Build history of the part. All positions in model axes, mm. Face numbers are marked on the shaded views. A direction names the side the tool comes from. Give positions to 0.01 mm unless a question says otherwise; leave off trailing zeros. Write each loop counter-clockwise with the first axis right and the second up, starting at its lowest first coordinate (ties: lowest second). Pieces come first, ordered by that corner, then holes. Notation, with made-up numbers: (78.25, 6.5) -> (133.25, 6.5) arc R14 ccw to (133.25, 12.5) -> close; hole circle Ø1 at (-18, 10). An arc over 180 degrees is marked (long way). One line per question, with ' | ' between items. Start each with the question number.
(1) Band-saw the part on C-C, the plane z = -3. Give the cut face in (x, y), and give its area (3 significant figures).
(2) Drill centre lines: probe 1 along X at (y, z) = (2.5, -2.25); probe 2 along X at (y, z) = (-2.5, -10.5). Where is each one in solid material? Low to high. Write a range as from..to.
(3) Band-saw the part on D-D, the plane x = 1.75. Give the cut face in (y, z).
(4) Band-saw the part on B-B, the plane y = 0. Give the cut face in (x, z).
(5) Band-saw the part on A-A, the plane x = 0. Give the cut face in (y, z), and give its area (3 significant figures).
(6) Tool access for the marked faces 1, 2 and 3: list every direction of +Z, -Z, +X, -X, +Y, -Y with a clear straight run to the whole face (end or side of a thin tool).
(7) Pin check, flat tips, straight feed: P1, Ø2, axis at x = -2.5, z = -8, coming from the +Y side; P2, Ø2, axis at x = -2, z = -9, coming from the -Y side; P3, Ø3, axis at x = 1, y = -1.5, coming from the -Z side. Stop position of each tip, or through.
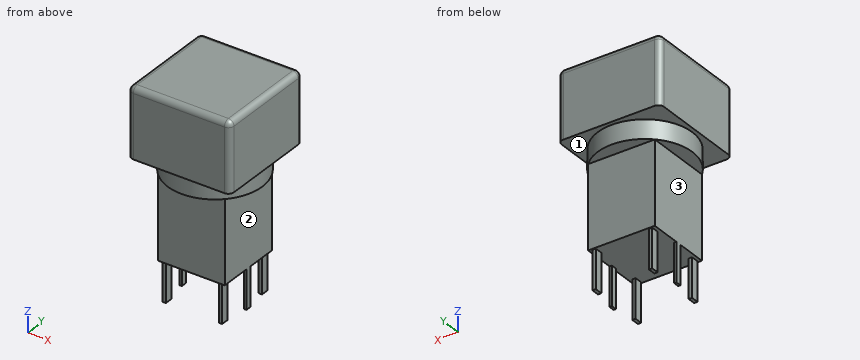
from build123d import *

# Parameters (mm, degrees)
SKETCH_1_W      = 9.2
SKETCH_1_H      = 9.2
EXTRUDE_1_DEPTH = 6.2
FILLET_1_R      = 0.5
SKETCH_2_R      = 4.25
EXTRUDE_2_DEPTH = 1.7
SKETCH_3_W      = 6
SKETCH_3_H      = 6
EXTRUDE_3_DEPTH = 7.45
SKETCH_4_W      = 0.3
SKETCH_4_H      = 0.7
SKETCH_4_W_2    = 0.2
SKETCH_4_H_2    = 0.5
EXTRUDE_4_DEPTH = 3.5


with BuildPart() as part:
    # Эскиз1 → Бобышка-Вытянуть1 (new body)
    with BuildSketch(Plane.XY):
        Rectangle(SKETCH_1_W, SKETCH_1_H)
    extrude(amount=EXTRUDE_1_DEPTH)

    # Скругление1
    fillet_1_edges = [part.edges().sort_by_distance(p)[0] for p in [
        (-4.6, 0, 6.2),
        (0, -4.6, 6.2),
        (4.6, 0, 6.2),
        (4.6, -4.6, 3.1),
        (-4.6, -4.6, 3.1),
        (-4.6, 4.6, 3.1),
        (4.6, 4.6, 3.1),
        (0, 4.6, 6.2),
    ]]
    fillet(fillet_1_edges, radius=FILLET_1_R)

    # Эскиз2 → Бобышка-Вытянуть2 (add)
    with BuildSketch(Plane(origin=(0, 0, 0), x_dir=(-1, 0, 0), z_dir=(0, 0, -1))):
        Circle(SKETCH_2_R)
    extrude(amount=EXTRUDE_2_DEPTH)

    # Эскиз3 → Бобышка-Вытянуть3 (add)
    with BuildSketch(Plane(origin=(0, 0, -1.7), x_dir=(-1, 0, 0), z_dir=(0, 0, -1))):
        Rectangle(SKETCH_3_W, SKETCH_3_H)
    extrude(amount=EXTRUDE_3_DEPTH)

    # Эскиз4 → Бобышка-Вытянуть4 (add)
    with BuildSketch(Plane(origin=(0, 0, -9.15), x_dir=(-1, 0, 0), z_dir=(0, 0, -1))):
        with Locations((-2.54, 2.54)):
            Rectangle(SKETCH_4_W, SKETCH_4_H)
        with Locations((2.54, 2.54)):
            Rectangle(SKETCH_4_W, SKETCH_4_H)
        with Locations((2.54, -2.54)):
            Rectangle(SKETCH_4_W, SKETCH_4_H)
        with Locations((-2.54, -2.54)):
            Rectangle(SKETCH_4_W, SKETCH_4_H)
        with Locations((2.9, 0)):
            Rectangle(SKETCH_4_W_2, SKETCH_4_H_2)
        with Locations((-2.9, 0)):
            Rectangle(SKETCH_4_W_2, SKETCH_4_H_2)
    extrude(amount=EXTRUDE_4_DEPTH)


solid = part.part
Results:
1) outline: (-3, -3) -> (3, -3) -> (3, 3) -> (-3, 3) -> close | area: 36.0 mm²
2) probe 1: x = -3..3 | probe 2: x = -2.69..-2.39, 2.39..2.69
3) outline: (-4.6, 0) -> (-3.87, 0) -> (-3.87, -1.7) -> (-3, -1.7) -> (-3, -9.15) -> (3, -9.15) -> (3, -1.7) -> (3.87, -1.7) -> (3.87, 0) -> (4.6, 0) -> (4.6, 5.7) arc R0.5 ccw to (4.1, 6.2) -> (-4.1, 6.2) arc R0.5 ccw to (-4.6, 5.7) -> close
4) outline: (-4.6, 0) -> (-4.25, 0) -> (-4.25, -1.7) -> (-3, -1.7) -> (-3, -12.65) -> (-2.8, -12.65) -> (-2.8, -9.15) -> (2.8, -9.15) -> (2.8, -12.65) -> (3, -12.65) -> (3, -1.7) -> (4.25, -1.7) -> (4.25, 0) -> (4.6, 0) -> (4.6, 5.7) arc R0.5 ccw to (4.1, 6.2) -> (-4.1, 6.2) arc R0.5 ccw to (-4.6, 5.7) -> close
5) outline: (-4.6, 0) -> (-4.25, 0) -> (-4.25, -1.7) -> (-3, -1.7) -> (-3, -9.15) -> (3, -9.15) -> (3, -1.7) -> (4.25, -1.7) -> (4.25, 0) -> (4.6, 0) -> (4.6, 5.7) arc R0.5 ccw to (4.1, 6.2) -> (-4.1, 6.2) arc R0.5 ccw to (-4.6, 5.7) -> close | area: 116 mm²
6) face 1: -Z | face 2: -Z, +X, +Y, -Y | face 3: -Z, -X, +Y, -Y
7) P1: stops at y = 3 | P2: stops at y = -3 | P3: stops at z = -9.15
